Check sheet for the modelled part. Datum: model origin and axes. Units: mm. A direction names the side the tool comes from. Give positions to 0.01 mm unless a question says otherwise; leave off trailing zeros. Loops run counter-clockwise (first coordinate to the right, second up) from the corner with the lowest first, then second, coordinate; pieces in that order, holes last. Notation, with made-up numbers: M 89,15 L 97,15 A23 ccw 97,48 Z; hole C -10,11.25 d10. An arc over 180 degrees is marked long. Put each result on its own line as item: value. Start each with the question number.
```python
from build123d import *

# Parameters (mm, degrees)
SKETCH1_W           = 3.175
SKETCH1_H           = 5
BOSS_EXTRUDE1_DEPTH = 3.175


with BuildPart() as part:
    # Sketch1 → Boss-Extrude1 (new body)
    with BuildSketch(Plane(origin=(0, 0, 0), x_dir=(1, 0, 0), z_dir=(0, 1, 0))):
        Polygon((-104.648, -5), (-101.473, -5), (-101.473, -10), (-104.648, -10), (-104.648, -15), (-101.473, -15), (-101.473, -20), (-104.648, -20), (-104.648, -25), (-101.473, -25), (-101.473, -30), (-104.648, -30), (-104.648, -38.1), (-101.473, -38.1), (-3.175, -38.1), (0, -38.1), (0, -30), (-3.175, -30), (-3.175, -25), (0, -25), (0, -20), (-3.175, -20), (-3.175, -15), (0, -15), (0, -10), (-3.175, -10), (-3.175, -5), (0, -5), (0, 0), (0, 3.175), (0, 13.175), (-104.648, 13.175), (-104.648, 3.175), (-104.648, 0), align=None)
        with Locations((-80.186500028, -7.5)):
            Rectangle(SKETCH1_W, SKETCH1_H, mode=Mode.SUBTRACT)
        with Locations((-80.186500028, -17.5)):
            Rectangle(SKETCH1_W, SKETCH1_H, mode=Mode.SUBTRACT)
        with Locations((-80.186500028, -27.5)):
            Rectangle(SKETCH1_W, SKETCH1_H, mode=Mode.SUBTRACT)
        with Locations((-10.9855, -27.5)):
            Rectangle(SKETCH1_W, SKETCH1_H, mode=Mode.SUBTRACT)
        with Locations((-10.9855, -17.5)):
            Rectangle(SKETCH1_W, SKETCH1_H, mode=Mode.SUBTRACT)
        with Locations((-10.9855, -7.5)):
            Rectangle(SKETCH1_W, SKETCH1_H, mode=Mode.SUBTRACT)
    extrude(amount=BOSS_EXTRUDE1_DEPTH)


solid = part.part
```
Q1. Thickness scan on line 1 along X through (y, z) = (2, 28.5) (3 decimals). Record the ranges inside material, lowest first. Write a range as [from, to].
Q2. Mould release check, pull along X, two halves, no side actions. Record for faces 1 (the face through (-78.599, 2, 18)), 2 (the face through (0, 2, 23)), 3 (the face through (-78.599, 2, 8)), 4 (the face through (-104.648, 2, -4)): pulls with the +X half, pulls with the -X half, needs draft (parallel to the pull), parting line crosses it, or undercut.
Q3. Access from +Z, -Z, +X, -X, +Y, -Y to the whole of each face (thin tool, end or side, straight path). Record for faces 5 (the face through (-53, 3.175, 12)), 6 (the face through (-3.175, 2, 8)), 7 (the face through (-80, 2, 30)), 8 (the face through (0, 2, 34)), 9 (the face through (-103, 2, 10)).
Q4. Section check B-B, the plane y = 0.95. Give the number of separate pieces and of enclosed holes in the cut face, then the cut area to 3 significant figures.
Q5. Section check A-A, the plane z = 9. Record the cut outline in (x, y) (3 decimals), then the cut area to 3 significant figures.
Q6. Depth check by flat-ended pin: P1, Ø1.6, axis at y = 2.5, z = 27, coming from the -X side. Enter the tip coordinate at first touch or a pass-through.
Found:
1. line 1: x = [-101.473, -81.774], [-78.599, -12.573], [-9.398, -3.175]
2. face 1: undercut
2. face 2: pulls with the +X half
2. face 3: undercut
2. face 4: pulls with the -X half
3. face 5: +Z, -Z, +X, -X, +Y
3. face 6: +X, +Y, -Y
3. face 7: +Y, -Y
3. face 8: +Z, -Z, +X, +Y, -Y
3. face 9: -X, +Y, -Y
4. separate pieces: 1
4. enclosed holes: 6
4. area: 5,180 mm^2
5. outline: M -101.473,0 L -81.774,0 L -81.774,3.175 L -101.473,3.175 Z; M -78.599,0 L -12.573,0 L -12.573,3.175 L -78.599,3.175 Z; M -9.398,0 L -3.175,0 L -3.175,3.175 L -9.398,3.175 Z
5. area: 292 mm^2
6. P1: stops at x = -101.47
